from build123d import *

# Parameters (mm, degrees)
F0_W      = 31.75
F0_H      = 31.75
F1_DEPTH  = 9.525
F7_R      = 1.27
F11_DEPTH = 6.35
F12_R     = 3.1749
F14_DEPTH = 4.8006
F15_W     = 33.3248
F15_H     = 31.75
F16_DEPTH = 2.3876
F17_R     = 2.3876
F18_DEPTH = 12.7
F19_R     = 3.175
F20_R     = 1.27


# Not quite as in the source:
# - a fillet or chamfer is up to 0.001 mm smaller than in the source, because OpenCascade refuses the exact size


with BuildPart() as f1:
    # F0 (on Right) → F1 (new body)
    with BuildSketch(Plane.YZ):
        Rectangle(F0_W, F0_H)
    extrude(amount=F1_DEPTH)

    # F6: sweep along a path in F5
    with BuildLine(Plane.XZ.offset(12.7)) as f6_path:
        Line((9.525, 9.525), (15.875, 9.525))
        ThreePointArc((15.875, 9.525), (19.4783384003, 10.4308096264), (22.225, 12.9328865162))
        Line((22.225, 12.9328865162), (23.5505334947, 14.9312034475))
    # F2 (on face) → F6 (sweep)
    with BuildSketch(Plane.YZ.offset(9.525)):
        with BuildLine():
            ThreePointArc((-15.875, 12.7), (-12.7, 9.525), (-9.525, 12.7))
            ThreePointArc((-9.525, 12.7), (-10.4549359718, 14.9450640323), (-12.7000000057, 15.875))
            ThreePointArc((-12.7000000057, 15.875), (-14.9450640323, 14.9450640282), (-15.875, 12.7))
        make_face()
    sweep(path=f6_path.line)

    # F7
    f7_edges = [f1.edges().sort_by_distance(p)[0] for p in [
        (20.9047, -15.875, 16.686251),
    ]]
    fillet(f7_edges, radius=F7_R)

    # F10: F1 across plane


with BuildPart() as f1_1:
    add(f1.part)
    add(f1.part.mirror(Plane(origin=(0, 0, 15.875), x_dir=(1, 0, 0), z_dir=(0, -1, 0))))

    # F2 (on face) → F11 (join)
    with BuildSketch(Plane.YZ.offset(9.525)):
        with BuildLine():
            ThreePointArc((-9.525, -12.7), (-12.7, -9.525), (-15.875, -12.7))
            ThreePointArc((-15.875, -12.7), (-14.9450640303, -14.9450640303), (-12.7, -15.875))
            ThreePointArc((-12.7, -15.875), (-10.4549359697, -14.9450640303), (-9.525, -12.7))
        make_face()
        with BuildLine():
            ThreePointArc((12.7, -15.875), (14.9450640303, -14.9450640303), (15.875, -12.7))
            ThreePointArc((15.875, -12.7), (10.4549359697, -10.4549359697), (12.7, -15.875))
        make_face()
    extrude(amount=F11_DEPTH)

    # F12 (radius 3.175 in the source; OpenCascade refuses exactly that, so slightly less here)
    f12_edges = [f1_1.edges().sort_by_distance(p)[0] for p in [
        (4.7625, -15.875, 15.875),
        (4.7625, -15.875, -15.875),
        (4.7625, 15.875, -15.875),
        (4.7625, 15.875, 15.875),
    ]]
    fillet(f12_edges, radius=F12_R)

    # F13 (on face) → F14 (join)
    with BuildSketch(Plane(origin=(0, 0, 0), x_dir=(0, -1, 0), z_dir=(-1, 0, 0))):
        with BuildLine():
            Line((-12.7001, 15.875), (-24.5396645936, 15.875))
            Line((-24.5396645936, 15.875), (-24.5396645936, -15.875))
            Line((-24.5396645936, -15.875), (-12.7001, -15.875))
            ThreePointArc((-12.7001, -15.875), (-14.9450933196, -14.9450933196), (-15.875, -12.7001))
            Line((-15.875, -12.7001), (-15.875, 12.7001))
            ThreePointArc((-15.875, 12.7001), (-14.9450933196, 14.9450933196), (-12.7001, 15.875))
        make_face()
        with BuildLine():
            Line((12.7001, 15.875), (-12.7001, 15.875))
            ThreePointArc((-12.7001, 15.875), (-14.9450933196, 14.9450933196), (-15.875, 12.7001))
            Line((-15.875, 12.7001), (-15.875, -12.7001))
            ThreePointArc((-15.875, -12.7001), (-14.9450933196, -14.9450933196), (-12.7001, -15.875))
            Line((-12.7001, -15.875), (12.7001, -15.875))
            ThreePointArc((12.7001, -15.875), (14.9450933196, -14.9450933196), (15.875, -12.7001))
            Line((15.875, -12.7001), (15.875, 12.7001))
            ThreePointArc((15.875, 12.7001), (14.9450933196, 14.9450933196), (12.7001, 15.875))
        make_face()
        with BuildLine():
            Line((24.5396645936, 15.875), (12.7001, 15.875))
            ThreePointArc((12.7001, 15.875), (14.9450933196, 14.9450933196), (15.875, 12.7001))
            Line((15.875, 12.7001), (15.875, -12.7001))
            ThreePointArc((15.875, -12.7001), (14.9450933196, -14.9450933196), (12.7001, -15.875))
            Line((12.7001, -15.875), (24.5396645936, -15.875))
            Line((24.5396645936, -15.875), (24.5396645936, 15.875))
        make_face()
    extrude(amount=F14_DEPTH)

    # F15 (on face) → F16 (cut)
    with BuildSketch(Plane(origin=(-4.8006, 0, 0), x_dir=(0, -1, 0), z_dir=(-1, 0, 0))):
        Rectangle(F15_W, F15_H)
    extrude(amount=-F16_DEPTH, mode=Mode.SUBTRACT)

    # F17 (on face) → F18 (join)
    with BuildSketch(Plane(origin=(-2.413, 0, 0), x_dir=(0, -1, 0), z_dir=(-1, 0, 0))):
        with Locations((0, 11.0998)):
            Circle(F17_R)
    extrude(amount=F18_DEPTH)

    # F19
    f19_edges = [f1_1.edges().sort_by_distance(p)[0] for p in [
        (-2.4003, 24.539665, 15.875),
        (-2.4003, 24.539665, -15.875),
        (-2.4003, -24.539665, -15.875),
        (-2.4003, -24.539665, 15.875),
    ]]
    fillet(f19_edges, radius=F19_R)

    # F20
    f20_edges = [f1_1.edges().sort_by_distance(p)[0] for p in [
        (-15.113, 2.3876, 11.0998),
    ]]
    fillet(f20_edges, radius=F20_R)


solid = f1_1.part
Geometry check sheet. Reference: the model listing, model coordinates, mm. A direction names the side the tool comes from. Give positions to 0.01 mm unless a question says otherwise; leave off trailing zeros. Write each loop counter-clockwise with the first axis right and the second up, starting at its lowest first coordinate (ties: lowest second). Pieces come first, ordered by that corner, then holes. Notation, with made-up numbers: (75.5, 41) - (94.5, 41) arc R23 ccw to (94.5, 74) - close; hole circle Ø1 at (73, -35). An arc over 180 degrees is marked (long way). Put each result on its own line as item: value.
1. Sectioned sample at A-A, the plane x = 13.5. Enter the section's corners in (y, z) (3 decimals), plus the area to 3 significant figures.
Ans:
outline: circle Ø6.35 at (-12.7, -12.7); circle Ø6.35 at (-12.7, 12.7); circle Ø6.35 at (12.7, -12.7); circle Ø6.35 at (12.7, 12.7)
area: 127 mm²
2. Draft check along Y on faces 1 (the cylindrical face through (4.83, -14.97, -14.92)), 2 (the flat face through (0, -20, 0)), 3 (the cylindrical face through (4.83, 14.97, -14.92)), 4 (the flat face through (-2.413, 0, 0)). Enter one of: +Y half, -Y half, draft (parallel to the pull), parting line (faces both ways), or undercut.
Ans:
face 1: -Y half
face 2: draft
face 3: +Y half
face 4: undercut
3. Sectioned sample at C-C, the plane x = 7.5. Enter the section's corners in (y, z) (3 decimals), plus the area to 3 significant figures.
Ans:
outline: (-15.875, -12.7) arc R3.175 ccw to (-12.7, -15.875) - (12.7, -15.875) arc R3.175 ccw to (15.875, -12.7) - (15.875, 12.7) arc R3.175 ccw to (12.7, 15.875) - (-12.7, 15.875) arc R3.175 ccw to (-15.875, 12.7) - close
area: 999 mm²
4. Thickness scan on line 1 (Y direction, x = -4, z = 10.5); line 2 (Y direction, x = -4, z = 12.5); line 3 (X direction, y = 1.5, z = 1) (3 decimals). Record the ranges inside material, lowest first.
Ans:
line 1: y = -24.54 to -16.66, -2.31 to 2.31, 16.66 to 24.54
line 2: y = -24.54 to -16.66, -1.93 to 1.93, 16.66 to 24.54
line 3: x = -2.413 to 9.525
5. Sectioned sample at B-B, the plane z = -4. Enter the section's corners in (x, y) (3 decimals), plus the area to 3 significant figures.
Ans:
outline: (-4.801, -24.54) - (0, -24.54) - (0, -15.875) - (9.525, -15.875) - (9.525, 15.875) - (0, 15.875) - (0, 24.54) - (-4.801, 24.54) - (-4.801, 16.662) - (-2.413, 16.662) - (-2.413, -16.662) - (-4.801, -16.662) - close
area: 458 mm²
6. Set-up check for faces 5 (the flat face through (5, 15.875, 0)), 6 (the cylindrical face through (4.83, 14.92, 14.97)), 7 (the flat face through (-4, 16.662, 0)), 8 (the cylindrical face through (-8.05, 0.52, 8.77)), 9 (the cylindrical face through (4.83, -14.97, 14.92)): record each of +Z, -Z, +X, -X, +Y, -Y from which the full face is reachable in a straight line by a thin tool's end or side.
Ans:
face 5: +Z, -Z, +X, +Y
face 6: +Z, +Y
face 7: +Z, -Z, -X
face 8: -X
face 9: +Z, -Y
7. Sectioned sample at D-D, the plane y = -18. Enter the section's corners in (x, z) (3 decimals), plus the area to 3 significant figures.
Ans:
outline: (-4.801, -15.875) - (0, -15.875) - (0, 15.875) - (-4.801, 15.875) - close
area: 152 mm²
8. Go/stop test with flat-tipped pins: pin 1 (4 mm diameter, centred on y = -20.5, z = 6.5, fed in from -X); pin 2 (1 mm diameter, centred on x = 13, z = 12, fed in from +Y); pin 3 (5 mm diameter, centred on y = 11.5, z = -13.5, fed in from +X) (3 decimals). Record where each tip stops, or that it passes through.
Ans:
pin 1: stops at x = -4.8
pin 2: stops at y = 15.87
pin 3: stops at x = 15.875
